Autodesk Inventor part; units mm, degrees
ref_plane "YZ Plane" through (0, 0, 0) normal (1, 0, 0) x (0, 1, 0)
ref_plane "XZ Plane" through (0, 0, 0) normal (0, 1, 0) x (-1, 0, 0)
ref_plane "XY Plane" through (0, 0, 0) normal (0, 0, 1) x (1, 0, 0)
sketch "Sketch1" plane through (0, 0, 0) normal (0, 1, 0) x (-1, 0, 0)
  line L0 (0, 0) -> (-244, 0)
  line L1 (-244, 0) -> (-244, -305)
  line L2 (-244, -305) -> (0, -305)
  line L3 (0, -305) -> (0, 0)
  dimension "d0" = 244
  dimension "d1" = 305
extrude "Extrusion1" add sketch "Sketch1" along normal blind 1.651
sketch "Sketch2" plane through (0, 1.651, 0) normal (0, 1, 0) x (1, 0, 0)
  line L0 (0, 305) -> (0, 0)
  line L1 (0, 0) -> (244, 0)
  line L2 (244, 0) -> (244, 305)
  point P0 (10, 17)
  point P1 (10, 96)
  point P2 (10, 142)
  point P3 (238, 17)
  point P4 (177.9993, 17)
  point P5 (176.1481, 141)
  point P6 (178, 298)
  point P7 (23, 298)
  point P8 (238, 141)
  point P9 (238, 298)
  dimension "d4" = 10
  dimension "d5" = 17
  dimension "d6" = 79
  dimension "d8" = 46
  dimension "d11" = 6
  dimension "d14" = 17
  dimension "d16" = 155
  dimension "d17" = 23
  dimension "d18" = 124
  dimension "d19" = 157
hole "Hole1" at (10, 1.651, -17) at (10, 1.651, -96) at (10, 1.651, -142) at (238, 1.651, -17) at (177.9993, 1.651, -17) at (176.1481, 1.651, -141) at (178, 1.651, -298) at (23, 1.651, -298) at (238, 1.651, -141) at (238, 1.651, -298) direction (0, -1, 0) diameter 4 end through all
properties part number "atxboard"
Input: part model. Units: mm. Frame: model coordinates. Coordinates: 2 decimals unless noted, no trailing zeros. Answer in a Markdown table with one row per item.
(1) Mould query, pull axis Y, two halves, no side actions, for faces 1 (the face through (124, 0, -150)), 2 (the face through (124, 1.651, -150)). Classes: pulls with the +Y half, pulls with the -Y half, needs draft (parallel to the pull), parting line crosses it, or undercut.
Model answer:
| item | result |
|---|---|
| face 1 | pulls with the -Y half |
| face 2 | pulls with the +Y half |
(2) Pin query (flat end, axial travel): P1, Ø4.5, axis at x = 178, z = -17, coming from the -Y side. Return the tip coordinate at first contact, or that it passes through.
Model answer:
| item | result |
|---|---|
| P1 | stops at y = 0 |
(3) Material intervals for L1, parallel to X at y = 1.15, z = -17; L2, parallel to Z at x = 238, y = 0.9; L3, parallel to X at y = 1, z = -298, sorted ascending. Write a range as from..to.
Model answer:
| item | result |
|---|---|
| L1 | x = 0..8, 12..176, 180..236, 240..244 |
| L2 | z = -305..-300, -296..-143, -139..-19, -15..0 |
| L3 | x = 0..21, 25..176, 180..236, 240..244 |
